from build123d import *

# Parameters (mm, degrees)
SKETCH010_R      = 18
SKETCH010_R_2    = 5
SKETCH010_R_3    = 2
EXTRUDE010_DEPTH = 5
SKETCH011_R      = 8
SKETCH011_R_2    = 5
EXTRUDE011_DEPTH = 8


with BuildPart() as extrude010:
    # Sketch010 (on Face29 of Cut003) → Extrude010 (new body)
    with BuildSketch(Plane.XY.offset(49)):
        Circle(SKETCH010_R)
        Circle(SKETCH010_R_2, mode=Mode.SUBTRACT)
        with Locations((8.485281, 8.485281)):
            Circle(SKETCH010_R_3, mode=Mode.SUBTRACT)
        with Locations((8.485281, -8.485281)):
            Circle(SKETCH010_R_3, mode=Mode.SUBTRACT)
        with Locations((-8.485281, -8.485281)):
            Circle(SKETCH010_R_3, mode=Mode.SUBTRACT)
        with Locations((-8.485281, 8.485281)):
            Circle(SKETCH010_R_3, mode=Mode.SUBTRACT)
    extrude(amount=EXTRUDE010_DEPTH)


with BuildPart() as flangemockup:
    # Sketch011 (on Face8 of Extrude010) → Extrude011 (new body)
    with BuildSketch(Plane.XY.offset(54)):
        Circle(SKETCH011_R)
        Circle(SKETCH011_R_2, mode=Mode.SUBTRACT)
    extrude(amount=EXTRUDE011_DEPTH)

    # Fusion002: union Extrude010
    add(extrude010.part)


solid = flangemockup.part
Can you work these out from the model? Positions are in its coordinate system, mm. A direction names the side the tool comes from. Give positions to 0.01 mm unless a question says otherwise; leave off trailing zeros. Order: outer loops, then holes, each group sorted by start corner. A loop starts at its lowest first (then second) coordinate and runs counter-clockwise, first axis right, second up. Notation, with made-up numbers: M 48.25,6.5 L 74.25,6.5 A28 cw 74.25,24.5 Z; hole C 66.25,16.5 d3. An arc over 180 degrees is marked long. Use one line per item in the form item = value.
Item 1: Thinking about a two-plate mould opening in X: for faces 1 (the cylindrical face through (-1.73, -7.81, 57.94)), 2 (the flat face through (5.2, 0.1, 62)), 3 (the cylindrical face through (-1.08, -4.88, 55.41)), which applies, pulls with the +X half, pulls with the -X half, needs draft (parallel to the pull), parting line crosses it, or undercut?
Values follow:
face_1 = parting line crosses it
face_2 = needs draft
face_3 = undercut
Item 2: For faces 4 (the flat face through (8, -4, 54)), 5 (the cylindrical face through (-2.343, 17.847, 51.465)), which set-ups out of +Z, -Z, +X, -X, +Y, -Y let a thin tool reach every point of the face, with its end or its side?
Values follow:
face_4 = +Z
face_5 = +Z, -Z
Item 3: Will these pins go through, and if not, where does the flat tip stop? pin 1 Ø2 at (y, z) = (0.5, 52) entering from +X; pin 2 Ø2.5 at (x, y) = (-8.49, -8.49) entering from -Z; pin 3 Ø5 at (x, z) = (-13.5, 51.5) entering from +Y; pin 4 Ø5 at (y, z) = (1.5, 57) entering from -X.
Values follow:
pin_1 = 18
pin_2 = through
pin_3 = 14.25
pin_4 = -8
Item 4: If I drill on line 1 along Z through (x, y) = (-7, -14.5); line 2 along Y through (x, z) = (8.5, 53.25); line 3 along Y through (x, z) = (3.5, 60.75), over which ranges is the centre line in solid material (lowest first)? Write a range as [from, to].
Values follow:
line_1 = [49, 54]
line_2 = [-15.87, -10.49], [-6.49, 6.49], [10.49, 15.87]
line_3 = [-7.19, -3.57], [3.57, 7.19]
Item 5: If we section it at A-A, the plane y = 0: Write out the boundary of the cut face in (x, z).
Values follow:
outline = M -18,49 L -5,49 L -5,62 L -8,62 L -8,54 L -18,54 Z; M 5,49 L 18,49 L 18,54 L 8,54 L 8,62 L 5,62 Z
Item 6: If we section it at C-C, the plane z = 60.5: Write out the boundary of the cut face in (x, y), and give its area (3 significant figures).
Values follow:
outline = C 0,0 d16; hole C 0,0 d10
area = 123 mm^2
Item 7: If we section it at D-D, the plane y = -7.5: Write out the boundary of the cut face in (x, z).
Values follow:
outline = M -16.36,49 L -10.23,49 L -10.23,54 L -16.36,54 Z; M -6.74,49 L 6.74,49 L 6.74,54 L 2.78,54 L 2.78,62 L -2.78,62 L -2.78,54 L -6.74,54 Z; M 10.23,49 L 16.36,49 L 16.36,54 L 10.23,54 Z
